```python
from build123d import *

# Parameters (mm, degrees)
F3_DEPTH = 12.7


with BuildPart() as f2:
    # F1 (on Right) → F2 (revolve)
    with BuildSketch(Plane.YZ):
        with BuildLine():
            Line((-4.7625, 15.875), (-4.7625, 19.05))
            Line((-4.7625, 19.05), (-9.525, 19.05))
            Line((-9.525, 19.05), (-9.525, 0))
            Line((-9.525, 0), (9.525, 0))
            Line((9.525, 0), (9.525, 19.05))
            Line((9.525, 19.05), (4.7615565856, 19.05))
            Line((4.7615565856, 19.05), (4.7615565856, 15.9697899354))
            ThreePointArc((4.7615565856, 15.9697899354), (0.0464539006, 11.2075257948), (-4.7625, 15.875))
        make_face()
    revolve(axis=Axis((0, 0, 0), (0, 1, 0)))

    # F0 (on Front) → F3 (cut, symmetric)
    with BuildSketch(Plane.XZ):
        Polygon((3.7394976935, 6.477), (-3.7394976935, 6.477), (-7.4789953871, 0), (-3.7394976935, -6.477), (3.7394976935, -6.477), (7.4789953871, 0), align=None)
    extrude(amount=F3_DEPTH, both=True, mode=Mode.SUBTRACT)


solid = f2.part
```
Can you work these out from the model? Positions are in its coordinate system, mm. A direction names the side the tool comes from. Round coordinates to 2 decimals unless told otherwise and drop trailing zeros. Loops run counter-clockwise (first coordinate to the right, second up) from the corner with the lowest first, then second, coordinate; pieces in that order, holes last. Notation, with made-up numbers: M 18.5,-34.5 L 55.5,-34.5 A17 ccw 55.5,-20.5 Z; hole C -24,-4 d10. An arc over 180 degrees is marked long. Write item = value, one per line. Start each with the question number.
(1) Suppose I cut it at A-A on y = -5.25. Write out the boundary of the cut face in (x, z), plus the area to 3 significant figures.
(2) I'm going to push flat-ended pins straight in: P1, Ø6, axis at y = 1, z = 4.5, coming from the -X side; P2, Ø8, axis at x = -5, y = -7.5, coming from the +Z side; P3, Ø2, axis at x = 1.5, y = -2.5, coming from the +Z side. Where does each tip first touch, or does it pass through?
(3) If we mould it in two halves opening along X, with no side actions, what happens to faces 1 (the face through (-5.635, -0.133, -3.193)), 2 (the face through (-5.583, -0.133, 3.284)), 3 (the face through (0, 9.525, -8)), 4 (the face through (-11.59, -7.18, -15.12))? For each: released by +X, released by -X, zero draft, split by the parting line, or undercut.
(4) I need wall thicknesses on line 1 along Y through (x, z) = (-1, 16) (1 decimal); line 2 along Y through (x, z) = (14, -0.5) (3 decimals); line 3 along Z through (x, y) = (3.5, -6.5). Which ranges of each line are inside material? Lowest first, please.
(5) Which directions (+Z, -Z, +X, -X, +Y, -Y) give clear straight access to the entire face, cutting with the end or side of a thin tool? Please do faces 5 (the face through (0, -9.525, 8)), 6 (the face through (16, -4.762, 4)), 7 (the face through (5.583, -0.133, -3.284)).
Answer block:
q1.outline = C 0,0 d38.1; hole M -7.48,0 L -3.74,-6.48 L 3.74,-6.48 L 7.48,0 L 3.74,6.48 L -3.74,6.48 Z
q1.area = 995 mm²
q2.P1 = -12.71
q2.P2 = 19.02
q2.P3 = 12.66
q3.face_1 = undercut
q3.face_2 = undercut
q3.face_3 = zero draft
q3.face_4 = split by the parting line
q4.line_1 = -9.5 to -4.8, 4.8 to 9.5
q4.line_2 = -9.525 to -4.341, 4.339 to 9.525
q4.line_3 = -18.73 to -6.48, 6.48 to 18.73
q5.face_5 = +Z, -Z, +X, -X, -Y
q5.face_6 = none
q5.face_7 = +Y, -Y
